The listing builds one solid part. Answer for the finished solid, in the listing's coordinates (mm). A direction names the side the tool comes from. Give positions to 0.01 mm unless a question says otherwise; leave off trailing zeros. Write each loop counter-clockwise with the first axis right and the second up, starting at its lowest first coordinate (ties: lowest second). Pieces come first, ordered by that corner, then holes.
```python
from build123d import *

# Parameters (mm, degrees)
PAD_DEPTH       = 3
SKETCH001_R     = 18.140088
PAD001_DEPTH    = 18
SKETCH002_R     = 12.72475
PAD002_DEPTH    = 25
FILLET_R        = 5
SKETCH003_R     = 10.036661
POCKET_DEPTH    = 39
SKETCH004_R     = 15.342719
POCKET001_DEPTH = 15
SKETCH005_R     = 1.671602
POCKET002_DEPTH = 9
CHAMFER_SIZE    = 1
POCKET003_DEPTH = 24
FILLET001_R     = 2
FILLET002_R     = 1


with BuildPart() as part:
    # Sketch → Pad (new body)
    with BuildSketch(Plane.XY):
        with BuildLine():
            ThreePointArc((15.819927, 8.439493), (-17.930285, 0), (15.819927, -8.439493))
            Line((43.550961, -8.439493), (15.819927, -8.439493))
            Line((43.550961, 8.439493), (43.550961, -8.439493))
            Line((15.819927, 8.439493), (43.550961, 8.439493))
        make_face()
    extrude(amount=PAD_DEPTH)

    # Sketch001 (on Face6 of Pad) → Pad001 (join)
    with BuildSketch(Plane.XY):
        Circle(SKETCH001_R)
    extrude(amount=PAD001_DEPTH)

    # Sketch002 (on Face9 of Pad001) → Pad002 (join)
    with BuildSketch(Plane.XY.offset(18)):
        Circle(SKETCH002_R)
    extrude(amount=PAD002_DEPTH)

    # Fillet
    fillet_edges = [part.edges().sort_by_distance(p)[0] for p in [
        (-18.140088, 0, 18),
    ]]
    fillet(fillet_edges, radius=FILLET_R)

    # Sketch003 (on Face12 of Fillet) → Pocket (cut)
    with BuildSketch(Plane.XY.offset(43)):
        Circle(SKETCH003_R)
    extrude(amount=-POCKET_DEPTH, mode=Mode.SUBTRACT)

    # Sketch004 (on Face10 of Pocket) → Pocket001 (cut)
    with BuildSketch(Plane(origin=(0, 0, 0), x_dir=(1, 0, 0), z_dir=(0, 0, -1))):
        Circle(SKETCH004_R)
    extrude(amount=-POCKET001_DEPTH, mode=Mode.SUBTRACT)

    # Sketch005 (on Face3 of Pocket001) → Pocket002 (cut)
    with BuildSketch(Plane.XY.offset(3)):
        with Locations((30.484385, 0)):
            Circle(SKETCH005_R)
    extrude(amount=-POCKET002_DEPTH, mode=Mode.SUBTRACT)

    # Chamfer
    chamfer_edges = [part.edges().sort_by_distance(p)[0] for p in [
        (28.812783, 0, 3),
    ]]
    chamfer(chamfer_edges, length=CHAMFER_SIZE)

    # Sketch006 → Pocket003 (cut)
    with BuildSketch(Plane.XZ):
        with BuildLine():
            ThreePointArc((5.267581, 5.153194), (0, 10.420775), (-5.267581, 5.153194))
            Line((-5.267581, 5.153194), (-5.267581, -7.655472))
            ThreePointArc((-5.267581, -7.655472), (0, -12.923053), (5.267581, -7.655472))
            Line((5.267581, -7.655472), (5.267581, 5.153194))
        make_face()
    extrude(amount=POCKET003_DEPTH, mode=Mode.SUBTRACT)

    # Fillet001
    fillet001_edges = [part.edges().sort_by_distance(p)[0] for p in [
        (43.550961, -8.439493, 1.5),
        (43.550961, 8.439493, 1.5),
    ]]
    fillet(fillet001_edges, radius=FILLET001_R)

    # Fillet002
    fillet002_edges = [part.edges().sort_by_distance(p)[0] for p in [
        (28.804144, -8.439493, 3),
        (28.804144, 8.439493, 3),
        (17.611702, -4.346347, 3),
        (17.611702, 4.346347, 3),
        (16.057327, -8.439493, 1.5),
        (42.965175, -7.853707, 3),
        (43.550961, 0, 3),
        (42.965175, 7.853707, 3),
        (16.057327, 8.439493, 1.5),
    ]]
    fillet(fillet002_edges, radius=FILLET002_R)


solid = part.part
```
Item 1: Which of the six approach directions +Z, -Z, +X, -X, +Y, -Y give full straight-line access (tool end or side, diameter ignored) to faces 4 (the face through (-2.76, -12.42, 30.32)), 5 (the face through (10, 3, 15)), 6 (the face through (29, 8.439, 1))?
Conclusion:
face 4: +Z
face 5: -Z
face 6: +Z, -Z, +X, +Y
Item 2: Each of these flat-tipped pins is pushed along its axis until it touches: P1, Ø12, axis at x = 31, z = 7, coming from the -Y side; P2, Ø3, axis at y = -16, z = 2, coming from the -X side; P3, Ø12, axis at x = 28, y = 0, coming from the +Z side. Where does it stop, or does it pass through?
Conclusion:
P1: stops at y = -8.44
P2: stops at x = -10.9
P3: stops at z = 3
Item 3: A cutting plane is placed at C-C, the plane z = 33.5. Give the vertices of the cut face in (x, y), plus the area to 3 significant figures.
Conclusion:
outline: circle Ø25.45 at (0, 0); hole circle Ø20.07 at (0, 0)
area: 192 mm2
Item 4: A cutting plane is placed at B-B, the plane y = 0. Give the vertices of the cut face in (x, z), plus the area to 3 significant figures.
Conclusion:
outline: (-18.14, 0) - (-15.34, 0) - (-15.34, 15) - (-10.04, 15) - (-10.04, 43) - (-12.72, 43) - (-12.72, 18) - (-13.14, 18) arc R5 ccw to (-18.14, 13) - close; (10.04, 15) - (15.34, 15) - (15.34, 0) - (28.81, 0) - (28.81, 2) - (27.81, 3) - (19.14, 3) arc R1 cw to (18.14, 4) - (18.14, 13) arc R5 ccw to (13.14, 18) - (12.72, 18) - (12.72, 43) - (10.04, 43) - close; (32.16, 0) - (43.55, 0) - (43.55, 2) arc R1 ccw to (42.55, 3) - (33.16, 3) - (32.16, 2) - close
area: 321 mm2
Item 5: A cutting plane is placed at A-A, the plane x = 0. Give the vertices of the cut face in (y, z).
Conclusion:
outline: (-18.14, 10.42) - (-15.34, 10.42) - (-15.34, 15) - (-10.04, 15) - (-10.04, 43) - (-12.72, 43) - (-12.72, 18) - (-13.14, 18) arc R5 ccw to (-18.14, 13) - close; (10.04, 15) - (15.34, 15) - (15.34, 0) - (18.14, 0) - (18.14, 13) arc R5 ccw to (13.14, 18) - (12.72, 18) - (12.72, 43) - (10.04, 43) - close
Item 6: A cutting plane is placed at D-D, the plane x = 24.5. Give the vertices of the cut face in (y, z), plus the area to 3 significant figures.
Conclusion:
outline: (-8.44, 0) - (8.44, 0) - (8.44, 2) arc R1 ccw to (7.44, 3) - (-7.44, 3) arc R1 ccw to (-8.44, 2) - close
area: 50.2 mm2
Item 7: Determine the mould class of faces 1 (the face through (33, 2, 3)), 2 (the face through (5.268, -16, 3)), 3 (the face through (-13.37, 12.26, 6.41)) for opening direction X: pulls with the +X half, pulls with the -X half, needs draft (parallel to the pull), parting line crosses it, or undercut.
Conclusion:
face 1: needs draft
face 2: undercut
face 3: parting line crosses it
Item 8: Consider probe 1 along Y at (x, z) = (0, 35.5); probe 2 along X at (y, z) = (0, 7); probe 3 along Z at (x, y) = (37, 4.5). Determine where each line is inside the solid, lowest interval first.
Conclusion:
probe 1: y = -12.72 to -10.04, 10.04 to 12.72
probe 2: x = -18.14 to -15.34, 15.34 to 18.14
probe 3: z = 0 to 3
